Read the model definition and answer for the solid it produces. Units are mm, in the model's axes. A direction names the side the tool comes from. Coordinates: 2 decimals unless noted, no trailing zeros. Order: outer loops, then holes, each group sorted by start corner. A loop starts at its lowest first (then second) coordinate and runs counter-clockwise, first axis right, second up. Notation, with made-up numbers: M 48.25,-34 L 72.25,-34 A26 cw 72.25,3 Z; hole C 47,2 d8. An arc over 180 degrees is marked long. Write each question's results on one line, items separated by ' | '.
```python
from build123d import *

# Parameters (mm, degrees)
F0_R     = 2.25
F1_DEPTH = 85
F3_W     = 8.2
F3_H     = 17.972744
F3_H_2   = 20.743802
F4_DEPTH = 25


with BuildPart() as f1:
    # F0 (on Right) → F1 (new body)
    with BuildSketch(Plane.YZ):
        Circle(F0_R)
    extrude(amount=F1_DEPTH)

    # F3 (on offset) → F4 (cut)
    with BuildSketch(Plane.XY.offset(1)):
        with Locations((4.1, -0.105816)):
            Rectangle(F3_W, F3_H)
        with Locations((80.9, -0.062075)):
            Rectangle(F3_W, F3_H_2)
    extrude(amount=F4_DEPTH, mode=Mode.SUBTRACT)


solid = f1.part
```
(1) The part is cut by section B-B, the plane x = 66.5. Write down the section's boundary in (y, z), then the cut area to 3 significant figures.
Conclusion:
outline: C 0,0 d4.5 | area: 15.9 mm²
(2) For faces 1 (the flat face through (4, 0, 1)), 2 (the flat face through (85, 0, 0)), 3 (the flat face through (81, 0, 1)), determine the directions among +Z, -Z, +X, -X, +Y, -Y from which every point of the face is accessible in a straight line to the end or side of a thin tool.
Conclusion:
face 1: +Z, -X, +Y, -Y | face 2: +Z, -Z, +X, +Y, -Y | face 3: +Z, +X, +Y, -Y
(3) Straight lines are drawn through the part: line 1 (X direction, y = 0.05, z = 2); line 2 (Y direction, x = 19, z = -0.2); line 3 (Z direction, x = 68.5, y = 0.3). For each, find the intervals that lie inside material, in ascending order.
Conclusion:
line 1: 8.2 to 76.8 | line 2: -2.24 to 2.24 | line 3: -2.23 to 2.23
(4) The part is cut by section C-C, the plane z = -1.15. Write down the section's boundary in (x, y).
Conclusion:
outline: M 0,-1.93 L 85,-1.93 L 85,1.93 L 0,1.93 Z
(5) Given pin 1 (0.6 mm diameter, centred on y = 0.5, z = 1.5, fed in from +X); pin 2 (1.5 mm diameter, centred on x = 69, z = 0.5, fed in from -Y), each flat-ended and moving along its own axis, determine where each tip first touches the part or whether it passes through.
Conclusion:
pin 1: x = 76.8 | pin 2: y = -2.25
(6) The part is cut by section A-A, the plane y = 0. Write down the section's boundary in (x, z), then the cut area to 3 significant figures.
Conclusion:
outline: M 0,-2.25 L 85,-2.25 L 85,1 L 76.8,1 L 76.8,2.25 L 8.2,2.25 L 8.2,1 L 0,1 Z | area: 362 mm²
